Work out the finished part from the listing and answer in its coordinate system (mm). Coordinates: 2 decimals unless noted, no trailing zeros. Write each loop counter-clockwise with the first axis right and the second up, starting at its lowest first coordinate (ties: lowest second). Pieces come first, ordered by that corner, then holes. Notation, with made-up numbers: (3.25, 52) - (32.25, 52) arc R9 cw to (32.25, 67) - close; hole circle Ø9 at (78, 87.5). An arc over 180 degrees is marked (long way). Use one line per item in the form item = value. Start each with the question number.
Item 1: Given pin 1 (12 mm diameter, centred on x = -26, y = -2.5, fed in from -Z); pin 2 (5.5 mm diameter, centred on x = 44.47, y = 0, fed in from +Z), each flat-ended and moving along its own axis, determine where each tip first touches the part or whether it passes through.
Item 2: Determine the mould class of faces 1 (the cylindrical face through (42.131, 2.146, 3.131)), 2 (the flat face through (11, 1, 6.35)), 3 (the cylindrical face through (-11.012, -49.592, 3.774)) for opening direction Y: released by +Y, released by -Y, zero draft, split by the parting line, or undercut.
Item 3: Consider probe 1 along Y at (x, z) = (43, 5.25); probe 2 along Y at (x, z) = (-45.5, 1); probe 3 along X at (y, z) = (4, 3.75). Determine where each line is inside the solid, lowest interval first.
Item 4: A cutting plane is placed at C-C (z = 3). Give the number of separate pieces and of enclosed holes in the cut face, then the cut area to 3 significant figures.
Item 5: A cutting plane is placed at A-A (y = 0). Write down the section's boundary in (x, z).
Item 6: A cutting plane is placed at B-B (x = 0). Write down the section's boundary in (y, z).
from build123d import *

# Parameters (mm, degrees)
F0_R     = 50.8
F1_DEPTH = 6.35
F2_R     = 4.7625
F2_R_2   = 3.175
F3_DEPTH = 25.4
F4_SIZE  = 1.27


# Not quite as in the source:
# - a length typed as a fraction of an inch, garbled in the dataset ("3 / 203.2 mm" for 3/8 in), is restored


with BuildPart() as f1:
    # F0 (on Top) → F1 (new body)
    with BuildSketch(Plane.XY):
        Circle(F0_R)
    extrude(amount=F1_DEPTH)

    # F2 (on Top) → F3 (cut)
    with BuildSketch(Plane.XY):
        Circle(F2_R)
        with Locations((-44.6634478867, 0)):
            Circle(F2_R_2)
        with Locations((44.4713458419, 0)):
            Circle(F2_R_2)
    extrude(amount=F3_DEPTH, mode=Mode.SUBTRACT)

    # F4
    f4_edges = [f1.edges().sort_by_distance(p)[0] for p in [
        (-50.8, 0, 0),
    ]]
    chamfer(f4_edges, length=F4_SIZE)


solid = f1.part
Answer:
q1.pin_1 = 0
q1.pin_2 = through
q2.face_1 = undercut
q2.face_2 = zero draft
q2.face_3 = split by the parting line
q3.probe_1 = -27.05 to -2.81, 2.81 to 27.05
q3.probe_2 = -21.98 to -3.06, 3.06 to 21.98
q3.probe_3 = -50.64 to -2.58, 2.58 to 50.64
q4.separate_pieces = 1
q4.enclosed_holes = 3
q4.area = 7,970 mm²
q5.outline = (-50.8, 1.27) - (-49.53, 0) - (-47.84, 0) - (-47.84, 6.35) - (-50.8, 6.35) - close; (-41.49, 0) - (-4.76, 0) - (-4.76, 6.35) - (-41.49, 6.35) - close; (4.76, 0) - (41.3, 0) - (41.3, 6.35) - (4.76, 6.35) - close; (47.65, 0) - (49.53, 0) - (50.8, 1.27) - (50.8, 6.35) - (47.65, 6.35) - close
q6.outline = (-50.8, 1.27) - (-49.53, 0) - (-4.76, 0) - (-4.76, 6.35) - (-50.8, 6.35) - close; (4.76, 0) - (49.53, 0) - (50.8, 1.27) - (50.8, 6.35) - (4.76, 6.35) - close
